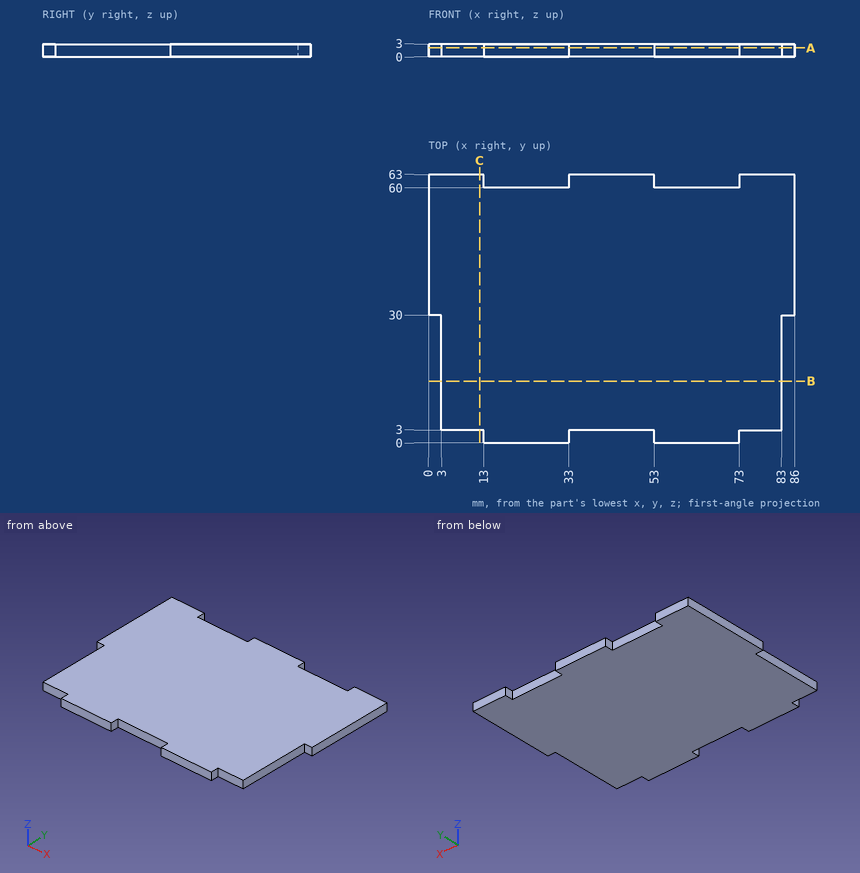
Drawing for the job (mm, zero at the part's lowest x, y, z). Give positions to 0.01 mm unless a question says otherwise; leave off trailing zeros. Write each loop counter-clockwise with the first axis right and the second up, starting at its lowest first coordinate (ties: lowest second). Pieces come first, ordered by that corner, then holes. Notation, with made-up numbers: M 51,-24 L 85,-24 A25 ccw 85,-4 Z; hole C -20.75,12.25 d11. An arc over 180 degrees is marked long. Return JSON: item names as keys, results as strings. Group by question number.
(1) Flat gauge pins, fed straight in: pin 1 Ø0.9 at (x, z) = (19, 1.5) entering from +Y; pin 2 Ø1.5 at (y, z) = (2, 1.5) entering from -X; pin 3 Ø1.5 at (y, z) = (1, 1.5) entering from +X. Where does each tip first touch, or does it go through?
(2) Band-saw the part on A-A (z = 2.1). Give the cut face in (x, y), and give its area (3 significant figures).
(3) Drill centre lines: L1, parallel to X at y = 60.5, z = 0.8; L2, parallel to Y at x = 24, z = 1.3; L3, parallel to X at y = 22, z = 2.75. Where is each one in solid material? Low to high. Write a range as [from, to].
(4) Band-saw the part on C-C (x = 12). Give the cut face in (y, z), and give its area (3 significant figures).
(5) Band-saw the part on B-B (y = 14.5). Give the cut face in (x, z), and give its area (3 significant figures).
Entries:
{
 "1": {"pin 1": "stops at y = 60", "pin 2": "stops at x = 13", "pin 3": "stops at x = 73"},
 "2": {"outline": "M 0,30 L 3,30 L 3,3 L 13,3 L 13,0 L 33,0 L 33,3 L 53,3 L 53,0 L 73,0 L 73,3 L 83,3 L 83,30 L 86,30 L 86,63 L 73,63 L 73,60 L 53,60 L 53,63 L 33,63 L 33,60 L 13,60 L 13,63 L 0,63 Z", "area": "5,000 mm^2"},
 "3": {"L1": "x = [0, 13], [33, 53], [73, 86]", "L2": "y = [0, 60]", "L3": "x = [3, 83]"},
 "4": {"outline": "M 3,0 L 63,0 L 63,3 L 3,3 Z", "area": "180 mm^2"},
 "5": {"outline": "M 3,0 L 83,0 L 83,3 L 3,3 Z", "area": "240 mm^2"}
}
